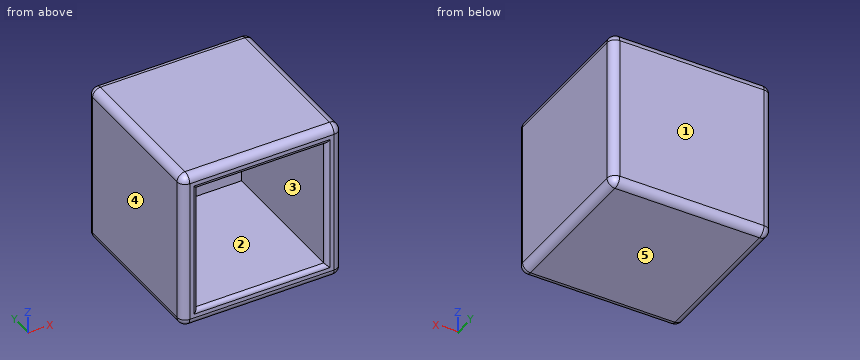
```python
from build123d import *

# Parameters (mm, degrees)
F0_W     = 20
F0_H     = 20
F1_DEPTH = 10
F2_T     = -2
F3_R     = 1
F4_R     = 0.5


with BuildPart() as f1:
    # F0 (on Front) → F1 (new body, symmetric)
    with BuildSketch(Plane.XZ):
        Rectangle(F0_W, F0_H)
    extrude(amount=F1_DEPTH, both=True)

    # F2
    f2_openings = [f1.faces().sort_by_distance(p)[0] for p in [
        (0, -10, 0),
    ]]
    offset(amount=F2_T, openings=f2_openings)

    # F3
    f3_edges = [f1.edges().sort_by_distance(p)[0] for p in [
        (0, -10, -10),
        (10, 10, 0),
        (10, 0, 10),
        (10, -10, 0),
        (10, 0, -10),
        (-10, 0, -10),
        (0, 10, -10),
        (-10, -10, 0),
        (-10, 0, 10),
        (-10, 10, 0),
        (0, 10, 10),
        (0, -10, 10),
    ]]
    fillet(f3_edges, radius=F3_R)

    # F4
    f4_edges = [f1.edges().sort_by_distance(p)[0] for p in [
        (-8, -10, 0),
        (0, -10, -8),
        (8, -10, 0),
        (0, -10, -9),
        (-9, -10, 0),
        (9, -10, 0),
        (0, -10, 9),
        (0, -10, 8),
    ]]
    fillet(f4_edges, radius=F4_R)


solid = f1.part
```
The model under review builds one solid part; all positions refer to its coordinate system, in mm. Face numbers are marked on the shaded views. A direction names the side the tool comes from. Give positions to 0.01 mm unless a question says otherwise; leave off trailing zeros. Write each loop counter-clockwise with the first axis right and the second up, starting at its lowest first coordinate (ties: lowest second). Pieces come first, ordered by that corner, then holes. Notation, with made-up numbers: M 48,75 L 81,75 A32 cw 81,112 Z; hole C 16,-32.75 d2. An arc over 180 degrees is marked long. Write each question's results on one line, items separated by ' | '. Start each with the question number.
1. Mouldability with a two-part tool opening along X and no side actions: class the marked faces 3, 4 and 5 as released by +X, released by -X, zero draft, split by the parting line, or undercut.
2. For probe 1 along X at (y, z) = (-6.75, 4.75); probe 2 along Y at (x, z) = (4.25, -1.5), list the stretches that pass through material, from the lowest coordinate up. Write a range as [from, to].
3. For the marked faces 1 and 2, list the 3-axis set-ups (+Z, -Z, +X, -X, +Y, -Y) from which the entire face can be reached by the end or side of a thin tool; tool diameter is ignored.
4. We need section B-B (z = 0.75). Write out the cut boundary in (x, y).
5. We need section C-C (y = 3). Write out the cut boundary in (x, z), and give its area (3 significant figures).
6. Insertion check: pin 1 Ø8 at (x, z) = (7.5, -0.5) entering from -Y. The pin has a flat end and moves straight along its axis. Give the tip position at first contact, or say it passes through.
7. We need section A-A (x = 0). Write out the cut boundary in (y, z), and give its area (3 significant figures).
Results found:
1) face 3: undercut | face 4: released by -X | face 5: zero draft
2) probe 1: x = [-10, -8], [8, 10] | probe 2: y = [8, 10]
3) face 1: +Z, -Z, +X, -X, +Y | face 2: -Y
4) outline: M -10,-9 A1 ccw -9,-10 L -8.5,-10 A0.5 ccw -8,-9.5 L -8,8 L 8,8 L 8,-9.5 A0.5 ccw 8.5,-10 L 9,-10 A1 ccw 10,-9 L 10,9 A1 ccw 9,10 L -9,10 A1 ccw -10,9 Z
5) outline: M -10,-9 A1 ccw -9,-10 L 9,-10 A1 ccw 10,-9 L 10,9 A1 ccw 9,10 L -9,10 A1 ccw -10,9 Z; hole M -8,-8 L 8,-8 L 8,8 L -8,8 Z | area: 143 mm^2
6) pin 1: stops at y = -10
7) outline: M -10,-9 A1 ccw -9,-10 L 9,-10 A1 ccw 10,-9 L 10,9 A1 ccw 9,10 L -9,10 A1 ccw -10,9 L -10,8.5 A0.5 ccw -9.5,8 L 8,8 L 8,-8 L -9.5,-8 A0.5 ccw -10,-8.5 Z | area: 111 mm^2
